from build123d import *

# Parameters (mm, degrees)
SKETCH1_W               = 21
SKETCH1_H               = 15
BOSS_EXTRUDE1_DEPTH     = 5
SKETCH2_W               = 3
SKETCH2_H               = 15
BOSS_EXTRUDE2_DEPTH     = 5
CUT_EXTRUDE1_DEPTH      = 18
SKETCH4_R               = 1.5
CUT_EXTRUDE2_DEPTH      = 19
CUT_EXTRUDE2_DEPTH_BACK = 4


with BuildPart() as part:
    # Sketch1 → Boss-Extrude1 (new body)
    with BuildSketch(Plane.XY):
        with Locations((-10.5, -7.5)):
            Rectangle(SKETCH1_W, SKETCH1_H)
    extrude(amount=BOSS_EXTRUDE1_DEPTH)

    # Sketch2 → Boss-Extrude2 (add)
    with BuildSketch(Plane.XY.offset(5)):
        with Locations((-1.5, -7.5)):
            Rectangle(SKETCH2_W, SKETCH2_H)
        with Locations((-19.5, -7.5)):
            Rectangle(SKETCH2_W, SKETCH2_H)
    extrude(amount=BOSS_EXTRUDE2_DEPTH)

    # Sketch3 → Cut-Extrude1 (cut)
    with BuildSketch(Plane(origin=(0, 0, 0), x_dir=(0, 0, -1), z_dir=(1, 0, 0))):
        with BuildLine():
            Line((-7.733661886, 0), (-10, 0))
            Line((-10, 0), (-10, -15))
            Line((-10, -15), (-7.733661886, -15))
            ThreePointArc((-7.733661886, -15), (-9.654849758, -7.5), (-7.733661886, 0))
        make_face()
    extrude(amount=-CUT_EXTRUDE1_DEPTH, mode=Mode.SUBTRACT)

    # Sketch4 → Cut-Extrude2 (cut, two sides)
    with BuildSketch(Plane(origin=(-18, 0, 0), x_dir=(0, 0, -1), z_dir=(1, 0, 0))) as cut_extrude2_sk:
        with Locations((-7.041389116, -7.762480296)):
            Circle(SKETCH4_R)
    extrude(amount=CUT_EXTRUDE2_DEPTH, mode=Mode.SUBTRACT)
    extrude(cut_extrude2_sk.sketch, amount=-CUT_EXTRUDE2_DEPTH_BACK, mode=Mode.SUBTRACT)


solid = part.part
Read the model definition and answer for the solid it produces. Units are mm, in the model's axes. A direction names the side the tool comes from. Coordinates: 2 decimals unless noted, no trailing zeros. Order: outer loops, then holes, each group sorted by start corner. A loop starts at its lowest first (then second) coordinate and runs counter-clockwise, first axis right, second up. Notation, with made-up numbers: (-4, 27) -> (1, 27) arc R25 ccw to (1, 61) -> close; hole circle Ø1 at (-31, -35). An arc over 180 degrees is marked (long way). Answer as a JSON object with one key per item and string values.
1) A cutting plane is placed at B-B, the plane z = 9.25. Determine the outline of the cut face in (x, y), plus the area to 3 significant figures.
Model answer:
{"outline": "(-21, -15) -> (-18, -15) -> (-18, 0) -> (-21, 0) -> close; (-3, -11.03) -> (0, -11.03) -> (0, -3.97) -> (-3, -3.97) -> close", "area": "66.2 mm²"}
2) This flat-tipped pin is pushed along its axis until it touches: pin 1 (1 mm diameter, centred on x = -3, y = -3.5, fed in from +Z). Where does it stop, or does it pass through?
Model answer:
{"pin 1": "stops at z = 9.26"}
3) A cutting plane is placed at D-D, the plane x = -16.75. Determine the outline of the cut face in (y, z).
Model answer:
{"outline": "(-15, 0) -> (0, 0) -> (0, 5) -> (-15, 5) -> close"}
4) Consider line 1 along X through (y, z) = (-3, 6); line 2 along Y through (x, z) = (-20, 7); line 3 along Z through (x, y) = (-13.5, -3.75). Determine where each line is inside the solid, lowest interval first. Write a range as from..to.
Model answer:
{"line 1": "x = -21..-18, -3..0", "line 2": "y = -15..-9.26, -6.26..0", "line 3": "z = 0..5"}
5) A cutting plane is placed at A-A, the plane y = -8.25. Determine the outline of the cut face in (x, z).
Model answer:
{"outline": "(-21, 0) -> (0, 0) -> (0, 5.62) -> (-3, 5.62) -> (-3, 5) -> (-18, 5) -> (-18, 5.62) -> (-21, 5.62) -> close; (-21, 8.46) -> (-18, 8.46) -> (-18, 10) -> (-21, 10) -> close; (-3, 8.46) -> (0, 8.46) -> (0, 9.64) -> (-3, 9.64) -> close"}
6) A cutting plane is placed at C-C, the plane y = -10.5. Determine the outline of the cut face in (x, z), plus the area to 3 significant figures.
Model answer:
{"outline": "(-21, 0) -> (0, 0) -> (0, 9.36) -> (-3, 9.36) -> (-3, 5) -> (-18, 5) -> (-18, 10) -> (-21, 10) -> close", "area": "133 mm²"}
7) A tool of negligible diameter and unlimited length cuts with its end or side. For faces 1 (the face through (-11, -7, 0)), 2 (the face through (-11, -7, 5)), from which of +Z, -Z, +X, -X, +Y, -Y can it reach the whole face along a straight path? Write none if from no direction.
Model answer:
{"face 1": "-Z, +X, -X, +Y, -Y", "face 2": "+Z, +Y, -Y"}
8) The mould has two halves that part along X. Classify faces 3 (the face through (-1.479, -7.61, 9.654)), 4 (the face through (-18, -8, 9)), 5 (the face through (-21, -8, 5)): released by +X, released by -X, zero draft, split by the parting line, or undercut.
Model answer:
{"face 3": "zero draft", "face 4": "undercut", "face 5": "released by -X"}
